```python
from build123d import *

# Parameters (mm, degrees)
BOSS_EXTRUDE1_DEPTH = 1


with BuildPart() as part:
    # Sketch1 → Boss-Extrude1 (new body)
    with BuildSketch(Plane(origin=(0, 0, 0), x_dir=(1, 0, 0), z_dir=(0, 1, 0))):
        with BuildLine():
            Line((0, 0), (25, 0))
            Line((25, 0), (25, 10))
            Line((25, 10), (23, 10))
            ThreePointArc((23, 10), (19.464466094, 11.464466094), (18, 15))
            Line((18, 15), (18, 20))
            Line((18, 20), (15, 20))
            Line((15, 20), (15, 16))
            Line((15, 16), (10, 16))
            Line((10, 16), (10, 20))
            Line((10, 20), (7, 20))
            Line((7, 20), (7, 15))
            ThreePointArc((7, 15), (5.535533906, 11.464466094), (2, 10))
            Line((2, 10), (0, 10))
            Line((0, 10), (0, 0))
        make_face()
        with BuildLine():
            Line((5, 7), (20, 7))
            ThreePointArc((20, 7), (22, 5), (20, 3))
            Line((20, 3), (5, 3))
            ThreePointArc((5, 3), (3, 5), (5, 7))
        make_face(mode=Mode.SUBTRACT)
    extrude(amount=BOSS_EXTRUDE1_DEPTH)


solid = part.part
```
Can you work these out from the model? Positions are in its coordinate system, mm. A direction names the side the tool comes from. Give positions to 0.01 mm unless a question says otherwise; leave off trailing zeros. Loops run counter-clockwise (first coordinate to the right, second up) from the corner with the lowest first, then second, coordinate; pieces in that order, holes last. Notation, with made-up numbers: M -38.5,42.5 L -11.5,42.5 A19 ccw -11.5,55.5 Z; hole C 43,55.5 d5. An arc over 180 degrees is marked long. Use CSV: the item, a comma, the result in double quotes. Start each with the question number.
1. Imagine slicing it at A-A, the plane x = 6. Write out the boundary of the cut face in (y, z), plus the area to 3 significant figures.
2. If I drill on L1, parallel to X at y = 0.25, z = -18.75; L2, parallel to Z at x = 12.5, y = 0.15; L3, parallel to X at y = 0.5, z = -5, over which ranges is the centre line in solid material (lowest first)?
3. For P1, Ø12, axis at x = 10.5, z = -14.5, coming from the -Y side; P2, Ø0.5, axis at x = 0.5, y = 0.5, coming from the -Z side; P3, Ø0.5, axis at y = 0.5, z = -18.5, coming from the -X side; P4, Ø0.5, axis at y = 0.5, z = -19, coming from the +X side, each with a flat end and sliding along its axis, tell me the tip position at first contact or that it passes through.
4. If we mould it in two halves opening along X, with no side actions, what happens to faces 4 (the face through (24, 0.5, -10)), 5 (the face through (12.5, 0.5, -16)), 6 (the face through (15, 0.5, -18)), 7 (the face through (0, 0.5, -5.1))? For each: released by +X, released by -X, zero draft, split by the parting line, or undercut.
5. Imagine slicing it at D-D, the plane z = -11.5. Write out the boundary of the cut face in (x, y), plus the area to 3 significant figures.
6. On a 3-axis mill with a long thin cutter (end or side, diameter ignored), from which of +Z, -Z, +X, -X, +Y, -Y can I reach the whole of each face in a straight line? I mean faces 1 (the face through (12.4, 0.5, -7)), 2 (the face through (10, 0.5, -18)), 3 (the face through (7, 0.5, -17.5)). Say none if no direction works.
7. Imagine slicing it at B-B, the plane y = 0.8. Write out the boundary of the cut face in (x, z).
8. Imagine slicing it at C-C, the plane z = -5.25. Write out the boundary of the cut face in (x, y).
Response values:
1,outline,"M 0,-12 L 1,-12 L 1,-7 L 0,-7 Z; M 0,-3 L 1,-3 L 1,0 L 0,0 Z"
1,area,"8.00 mm^2"
2,L1,"7 to 10, 15 to 18"
2,L2,"-16 to -7, -3 to 0"
2,L3,"0 to 3, 22 to 25"
3,P1,"y = 0"
3,P2,"z = -10"
3,P3,"x = 7"
3,P4,"x = 18"
4,face 4,"zero draft"
4,face 5,"undercut"
4,face 6,"undercut"
4,face 7,"released by -X"
5,outline,"M 5.57,0 L 19.43,0 L 19.43,1 L 5.57,1 Z"
5,area,"13.9 mm^2"
6,face 1,"+Y, -Y"
6,face 2,"-Z, +Y, -Y"
6,face 3,"-Z, -X, +Y, -Y"
7,outline,"M 0,-10 L 2,-10 A5 cw 7,-15 L 7,-20 L 10,-20 L 10,-16 L 15,-16 L 15,-20 L 18,-20 L 18,-15 A5 cw 23,-10 L 25,-10 L 25,0 L 0,0 Z; hole M 5,-7 L 20,-7 A2 ccw 20,-3 L 5,-3 A2 ccw Z"
8,outline,"M 0,0 L 3.02,0 L 3.02,1 L 0,1 Z; M 21.98,0 L 25,0 L 25,1 L 21.98,1 Z"
